from build123d import *

# Parameters (mm, degrees)
SKETCH1_R           = 5.715
BOSS_EXTRUDE1_DEPTH = 12.7
BOSS_EXTRUDE1_TAPER = 8
SKETCH2_R           = 2.3876
CUT_EXTRUDE1_DEPTH  = 10
FILLET1_R           = 1.27


with BuildPart() as part:
    # Sketch1 → Boss-Extrude1 (new body)
    with BuildSketch(Plane(origin=(0, 0, 0), x_dir=(1, 0, 0), z_dir=(0, 1, 0))):
        Circle(SKETCH1_R)
    extrude(amount=-BOSS_EXTRUDE1_DEPTH, taper=BOSS_EXTRUDE1_TAPER)

    # Sketch2 → Cut-Extrude1 (cut)
    with BuildSketch(Plane(origin=(0, 0, 0), x_dir=(1, 0, 0), z_dir=(0, 1, 0))):
        Circle(SKETCH2_R)
    extrude(amount=-CUT_EXTRUDE1_DEPTH, mode=Mode.SUBTRACT)

    # Fillet1
    fillet1_edges = [part.edges().sort_by_distance(p)[0] for p in [
        (-3.930131399, -12.7, 0),
    ]]
    fillet(fillet1_edges, radius=FILLET1_R)


solid = part.part
For this review, take the finished solid that the model builds, in its own axes (mm). A direction names the side the tool comes from. Coordinates: 2 decimals unless noted, no trailing zeros. Order: outer loops, then holes, each group sorted by start corner. A loop starts at its lowest first (then second) coordinate and runs counter-clockwise, first axis right, second up. Notation, with made-up numbers: (-19, 40) - (-15, 40) arc R24 ccw to (-15, 61) - close; hole circle Ø2 at (83, 80). An arc over 180 degrees is marked (long way). Answer as CSV lines item,"result". Start each with the question number.
1) Insertion check: P1, Ø4, axis at x = 4.5, y = -4, coming from the -Z side; P2, Ø1, axis at y = -8, z = 2, coming from the -X side; P3, Ø2, axis at y = -6, z = -1.5, coming from the -X side. Each pin has a flat end and moves straight along its axis. Give the tip position at first contact, or say it passes through.
2) Add section B-B (y = -9). State the section outline as (x, z) points, then the cut area to 3 significant figures.
3) To check wall thickness, follow line 1 along Z through (x, y) = (1.25, -7.5); line 2 along Z through (x, y) = (0, -7); line 3 along X through (y, z) = (-8.5, 0.75). State the ranges of each line that lie inside material, in increasing order. Write a range as [from, to].
4) Add section A-A (x = 0). State the section outline as (y, z) points (3 decimals).
5) Machinability: for faces 1 (the cylindrical face through (-0.52, -4.93, 2.33)), 2 (the flat face through (0, -12.7, 0)), which of the approach directions +Z, -Z, +X, -X, +Y, -Y give a long, thin tool a straight path to every point of the face, cutting with its end or side? Answer none if there is none.
6) Draft analysis for pull direction X (two halves, no side actions). For faces 3 (the conical face through (-0.613, -7.174, -4.667)), 4 (the flat face through (2.5, 0, 1.2)), 5 (the flat face through (0, -10, 0)), state which applies: +X half, -X half, draft (parallel to the pull), parting line (faces both ways), or undercut.
7) Add section C-C (y = -4). State the section outline as (x, z) points.
Result:
1,P1,"z = -4.55"
1,P2,"x = -4.35"
1,P3,"x = -4.91"
2,outline,"circle Ø8.9 at (0, 0); hole circle Ø4.78 at (0, 0)"
2,area,"44.3 mm^2"
3,line 1,"[-4.49, -2.03], [2.03, 4.49]"
3,line 2,"[-4.73, -2.39], [2.39, 4.73]"
3,line 3,"[-4.46, -2.27], [2.27, 4.46]"
4,outline,"(-12.7, -2.826) arc R1.27 ccw to (-11.607, -4.084) - (0, -5.715) - (0, -2.388) - (-10, -2.388) - (-10, 2.388) - (0, 2.388) - (0, 5.715) - (-11.607, 4.084) arc R1.27 ccw to (-12.7, 2.826) - close"
5,face 1,"+Y"
5,face 2,"+Z, -Z, +X, -X, -Y"
6,face 3,"parting line"
6,face 4,"draft"
6,face 5,"undercut"
7,outline,"circle Ø10.31 at (0, 0); hole circle Ø4.78 at (0, 0)"
